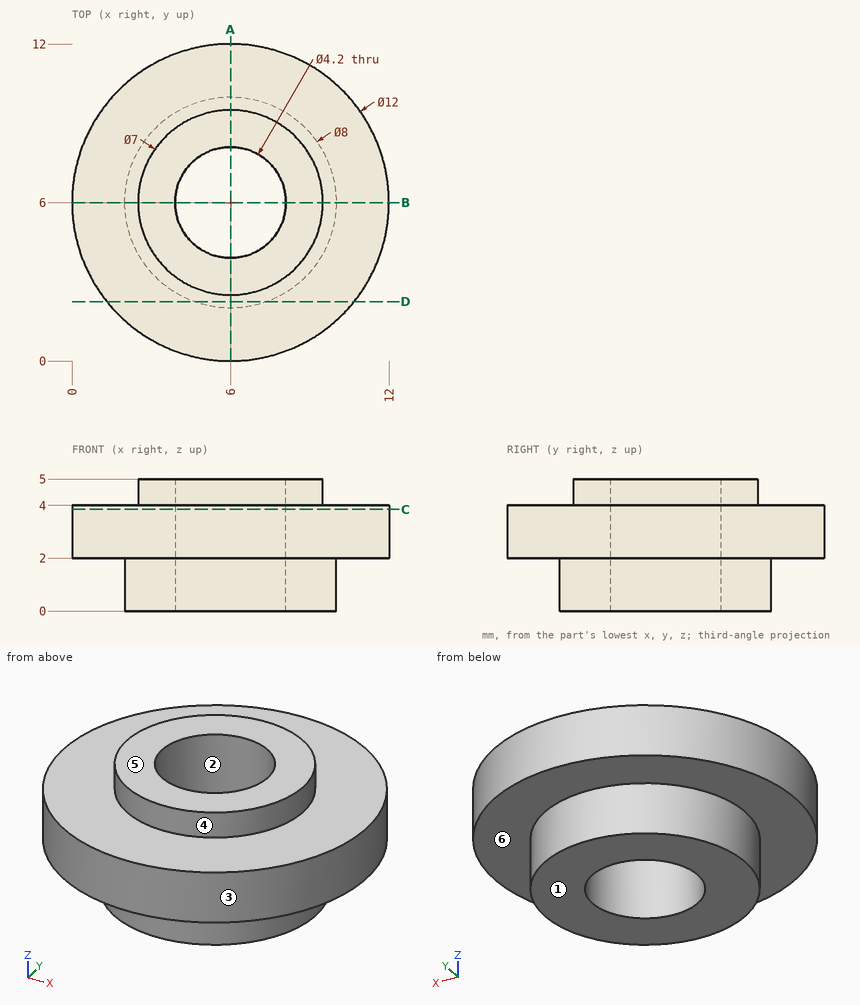
Geometry check sheet. Reference: drawing and pictorial views, mm from the part's lowest x, y, z. A direction names the side the tool comes from. Round coordinates to 2 decimals unless told otherwise and drop trailing zeros. Loops run counter-clockwise (first coordinate to the right, second up) from the corner with the lowest first, then second, coordinate; pieces in that order, holes last. Notation, with made-up numbers: (-19.75, 24) - (23.25, 24) arc R19 ccw to (23.25, 37) - close; hole circle Ø10 at (-14, 79.5). An arc over 180 degrees is marked (long way). Answer in a Markdown table with one row per item. Add a question column.
Q1. Material ranges on line 1 (Y direction, x = 6, z = 1.45); line 2 (Z direction, x = 2.75, y = 4.5); line 3 (Z direction, x = 3, y = 1.25), recorded low to high.
Q2. Gauge pin test, flat ends, axial feed: pin 1 (2 mm diameter, centred on x = 10.5, y = 2, fed in from +Z); pin 2 (1 mm diameter, centred on y = 2.5, z = 4, fed in from +X). Record the tip position at first contact, or that the pin passes through.
Q3. Tool access check on the marked faces 4, 5 and 6. Record the directions out of +Z, -Z, +X, -X, +Y, -Y that give a thin tool (end or side, any length) a straight path to the whole face; none if there is none.
Q4. Section check C-C on z = 3.85. Enter the section's corners in (x, y), plus the area to 3 significant figures.
Q5. Section check A-A on x = 6. Enter the section's corners in (y, z), plus the area to 3 significant figures.
Q6. Section check D-D on y = 2.25. Enter the section's corners in (x, z).
Q7. Release check for a two-part mould opening along Y. For the marked faces 1, 2 and 3 record: pulls with the +Y half, pulls with the -Y half, needs draft (parallel to the pull), parting line crosses it, or undercut.
Found:
| question | item | result |
|---|---|---|
| 1 | line 1 | y = 2 to 3.9, 8.1 to 10 |
| 1 | line 2 | z = 0 to 4 |
| 1 | line 3 | z = 2 to 4 |
| 2 | pin 1 | stops at z = 4 |
| 2 | pin 2 | stops at x = 11.2 |
| 3 | face 4 | +Z |
| 3 | face 5 | +Z, +X, -X, +Y, -Y |
| 3 | face 6 | -Z |
| 4 | outline | circle Ø12 at (6, 6); hole circle Ø4.2 at (6, 6) |
| 4 | area | 99.2 mm² |
| 5 | outline | (0, 2) - (2, 2) - (2, 0) - (3.9, 0) - (3.9, 5) - (2.5, 5) - (2.5, 4) - (0, 4) - close; (8.1, 0) - (10, 0) - (10, 2) - (12, 2) - (12, 4) - (9.5, 4) - (9.5, 5) - (8.1, 5) - close |
| 5 | area | 26.0 mm² |
| 6 | outline | (1.32, 2) - (4.61, 2) - (4.61, 0) - (7.39, 0) - (7.39, 2) - (10.68, 2) - (10.68, 4) - (1.32, 4) - close |
| 7 | face 1 | needs draft |
| 7 | face 2 | undercut |
| 7 | face 3 | parting line crosses it |
